Source: CAD feature listing. Evaluate the final solid. Frame: model axes, mm. A direction names the side the tool comes from. Coordinates: 2 decimals unless noted, no trailing zeros. Write each loop counter-clockwise with the first axis right and the second up, starting at its lowest first coordinate (ties: lowest second). Pieces come first, ordered by that corner, then holes. Notation, with made-up numbers: M 31.5,52.5 L 74.5,52.5 A18 ccw 74.5,81.5 Z; hole C 89,67 d2. An arc over 180 degrees is marked long. One line per item, written item: value. Start each with the question number.
Item 1: Cut plane C-C, the plane z = -15. Output: boundary loops of the cut face in (x, y), then the cut area to 3 significant figures.
Item 2: Mould query, pull axis X, two halves, no side actions, for faces 4 (the flat face through (-1, -1.524, -7)), 5 (the cylindrical face through (-41.86, 0.02, -7.84)), 6 (the cylindrical face through (-22.2, 0.02, -10.71)). Classes: released by +X, released by -X, zero draft, split by the parting line, or undercut.
Item 3: Pin query (flat end, axial travel): P1, Ø0.9, axis at x = 3, y = 1, coming from the -Z side; P2, Ø1, axis at x = -22, y = 1, coming from the -Z side. Return the tip coordinate at first contact, or that it passes through.
Item 4: Cut plane B-B, the plane x = 38. Output: boundary loops of the cut face in (y, z).
Item 5: Set-up query: faces 1 (the flat face through (17, 0, -9.901)), 2 (the cylindrical face through (51.045, -0.021, -4.914)), 3 (the flat face through (-48.217, 0.021, -4.079)). Return all of +Z, -Z, +X, -X, +Y, -Y with unobstructed straight access to the full face (end or side cutting, diameter ignored); none if empty.
Item 6: Cut plane D-D, the plane x = -33. Output: boundary loops of the cut face in (y, z).
Item 7: Cut plane A-A, the plane y = 0.1. Output: boundary loops of the cut face in (x, z).
Item 8: Ray query, L1, parallel to Z at x = 1.5, y = 0; L2, parallel to X at y = 0.9, z = -11.25; L3, parallel to X at y = 0.65, z = -16.5. Return the intervals inside material, ascending. Write a range as from..to.
```python
from build123d import *

# Parameters (mm, degrees)
F1_OUTLINE_DEPTH            = 1.524
F2_SLOT_DEPTH               = 58.881120617
F2_SLOT_DEPTH_BACK          = 58.881120617
F3A_HANDLEROUNDS_DEPTH      = 50.053367
F3A_HANDLEROUNDS_DEPTH_BACK = 11.2136936
F3B_ENDROUND_ANGLE          = 180
F4_RUNOUT_TOP_POS_ANGLE     = 90
F4_RUNOUT_BOT_POS_ANGLE     = 90
F4_RUNOUT_TOP_NEG_ANGLE     = 90
F4_RUNOUT_BOT_NEG_ANGLE     = 90


with BuildPart() as part:
    # SK_F1_Outline → F1_Outline (new, symmetric)
    with BuildSketch(Plane(origin=(0, 0, 0), x_dir=(1, 0, 0), z_dir=(0, 1, 0))):
        with BuildLine():
            Line((-34.3917778, 0), (50.053367, 0))
            ThreePointArc((50.053367, 0), (55.0037, 4.950333), (50.053367, 9.900666))
            Line((50.053367, 9.900666), (-17.8811936, 9.900666))
            ThreePointArc((-17.8811936, 9.900666), (-22.254213469, 10.732825234), (-26.01595, 13.1129786))
            ThreePointArc((-26.01595, 13.1129786), (-42.046618803, 17.559873613), (-54.849649, 6.9372734))
            ThreePointArc((-54.849649, 6.9372734), (-54.781279257, 5.257869905), (-53.4488136, 4.2333672))
            Line((-53.4488136, 4.2333672), (-49.0586522, 3.26009))
            Line((-49.0586522, 3.26009), (-47.3517722, 4.920488))
            Line((-47.3517722, 4.920488), (-48.8359196, 5.483987))
            ThreePointArc((-48.8359196, 5.483987), (-41.756588445, 7.823426138), (-35.8603296, 3.26009))
            Line((-35.8603296, 3.26009), (-34.3917778, 0))
        make_face()
    extrude(amount=F1_OUTLINE_DEPTH, both=True)

    # SK_F2_Slot → F2_Slot (cut, two sides: drawn at the far end of the back side and taken through both)
    with BuildSketch(Plane(origin=(0, 0, 0), x_dir=(1, 0, 0), z_dir=(0, 1, 0)).offset(-F2_SLOT_DEPTH_BACK)):
        with BuildLine():
            Line((48.7354118, 3.300222), (49.3954308, 3.300222))
            ThreePointArc((49.3954308, 3.300222), (51.0455418, 4.950333), (49.3954308, 6.600444))
            Line((49.3954308, 6.600444), (48.7354118, 6.600444))
            ThreePointArc((48.7354118, 6.600444), (47.0853008, 4.950333), (48.7354118, 3.300222))
        make_face()
    extrude(amount=F2_SLOT_DEPTH + F2_SLOT_DEPTH_BACK, mode=Mode.SUBTRACT)

    # SK_F3_StraightRounds → F3a_HandleRounds (cut, two sides: drawn at the far end of the back side and taken through both)
    with BuildSketch(Plane(origin=(0, 0, 0), x_dir=(0, 0, -1), z_dir=(1, 0, 0)).offset(-F3A_HANDLEROUNDS_DEPTH_BACK)):
        with BuildLine():
            Line((0, 1.127125), (-0.254, 1.127125))
            Line((-0.254, 1.127125), (-0.254, 1.778))
            Line((-0.254, 1.778), (0.396875, 1.778))
            Line((0.396875, 1.778), (0.396875, 1.524))
            ThreePointArc((0.396875, 1.524), (0.116241996, 1.407758004), (0, 1.127125))
        make_face()
        with BuildLine():
            Line((9.900666, 1.127125), (10.154666, 1.127125))
            Line((10.154666, 1.127125), (10.154666, 1.778))
            Line((10.154666, 1.778), (9.503791, 1.778))
            Line((9.503791, 1.778), (9.503791, 1.524))
            ThreePointArc((9.503791, 1.524), (9.784424004, 1.407758004), (9.900666, 1.127125))
        make_face()
        with BuildLine():
            Line((0, -1.127125), (-0.254, -1.127125))
            Line((-0.254, -1.127125), (-0.254, -1.778))
            Line((-0.254, -1.778), (0.396875, -1.778))
            Line((0.396875, -1.778), (0.396875, -1.524))
            ThreePointArc((0.396875, -1.524), (0.116241996, -1.407758004), (0, -1.127125))
        make_face()
        with BuildLine():
            Line((9.900666, -1.127125), (10.154666, -1.127125))
            Line((10.154666, -1.127125), (10.154666, -1.778))
            Line((10.154666, -1.778), (9.503791, -1.778))
            Line((9.503791, -1.778), (9.503791, -1.524))
            ThreePointArc((9.503791, -1.524), (9.784424004, -1.407758004), (9.900666, -1.127125))
        make_face()
    extrude(amount=F3A_HANDLEROUNDS_DEPTH + F3A_HANDLEROUNDS_DEPTH_BACK, mode=Mode.SUBTRACT)

    # SK_F3_EndRound → F3b_EndRound (revolve, symmetric, cut)
    with BuildSketch(Plane.XY.offset(-4.950333)) as f3b_endround_sk:
        with BuildLine():
            Line((55.0037, 1.127125), (55.2577, 1.127125))
            Line((55.2577, 1.127125), (55.2577, 1.778))
            Line((55.2577, 1.778), (54.606825, 1.778))
            Line((54.606825, 1.778), (54.606825, 1.524))
            ThreePointArc((54.606825, 1.524), (54.887458004, 1.407758004), (55.0037, 1.127125))
        make_face()
        with BuildLine():
            Line((55.0037, -1.127125), (55.2577, -1.127125))
            Line((55.2577, -1.127125), (55.2577, -1.778))
            Line((55.2577, -1.778), (54.606825, -1.778))
            Line((54.606825, -1.778), (54.606825, -1.524))
            ThreePointArc((54.606825, -1.524), (54.887458004, -1.407758004), (55.0037, -1.127125))
        make_face()
    revolve(axis=Axis((50.053367, -2.54, -4.950333), (0, 1, 0)), revolution_arc=F3B_ENDROUND_ANGLE / 2, mode=Mode.SUBTRACT)
    revolve(f3b_endround_sk.sketch, axis=Axis((50.053367, -2.54, -4.950333), (0, -1, 0)), revolution_arc=F3B_ENDROUND_ANGLE / 2, mode=Mode.SUBTRACT)

    # SK_F4_Runout1 → F4_Runout_Top_Pos (revolve, cut)
    with BuildSketch(Plane(origin=(0, 1.127125, 0), x_dir=(1, 0, 0), z_dir=(0, 1, 0))):
        Polygon((-11.2136936, 0), (-12.1460006, -0.164390878), (-12.1460006, -0.365125), (-11.2136936, -0.365125), align=None)
    revolve(axis=Axis((-9.9436936, 1.127125, -0.396875), (-1, 0, 0)), revolution_arc=F4_RUNOUT_TOP_POS_ANGLE, mode=Mode.SUBTRACT)

    # SK_F4_Runout2 → F4_Runout_Bot_Pos (revolve, cut)
    with BuildSketch(Plane(origin=(0, 1.127125, 0), x_dir=(1, 0, 0), z_dir=(0, 1, 0))):
        Polygon((-11.2136936, 9.900666), (-12.1460006, 10.065056878), (-12.1460006, 10.265791), (-11.2136936, 10.265791), align=None)
    revolve(axis=Axis((-9.9436936, 1.127125, -9.503791), (1, 0, 0)), revolution_arc=F4_RUNOUT_BOT_POS_ANGLE, mode=Mode.SUBTRACT)

    # SK_F4_Runout3 → F4_Runout_Top_Neg (revolve, cut)
    with BuildSketch(Plane(origin=(0, -1.127125, 0), x_dir=(1, 0, 0), z_dir=(0, 1, 0))):
        Polygon((-11.2136936, 0), (-12.1460006, -0.164390878), (-12.1460006, -0.365125), (-11.2136936, -0.365125), align=None)
    revolve(axis=Axis((-9.9436936, -1.127125, -0.396875), (1, 0, 0)), revolution_arc=F4_RUNOUT_TOP_NEG_ANGLE, mode=Mode.SUBTRACT)

    # SK_F4_Runout4 → F4_Runout_Bot_Neg (revolve, cut)
    with BuildSketch(Plane(origin=(0, -1.127125, 0), x_dir=(1, 0, 0), z_dir=(0, 1, 0))):
        Polygon((-11.2136936, 9.900666), (-12.1460006, 10.065056878), (-12.1460006, 10.265791), (-11.2136936, 10.265791), align=None)
    revolve(axis=Axis((-9.9436936, -1.127125, -9.503791), (-1, 0, 0)), revolution_arc=F4_RUNOUT_BOT_NEG_ANGLE, mode=Mode.SUBTRACT)


solid = part.part
```
From the geometry:
1. outline: M -48.16,-1.52 L -28.41,-1.52 L -28.41,1.52 L -48.16,1.52 Z
1. area: 60.2 mm²
2. face 4: zero draft
2. face 5: undercut
2. face 6: released by +X
3. P1: stops at z = -9.9
3. P2: stops at z = -10.83
4. outline: M -1.52,-9.5 A0.4 ccw -1.13,-9.9 L 1.13,-9.9 A0.4 ccw 1.52,-9.5 L 1.52,-0.4 A0.4 ccw 1.13,0 L -1.13,0 A0.4 ccw -1.52,-0.4 Z
5. face 1: -Z, +X, +Y, -Y
5. face 2: +Y, -Y
5. face 3: +Z, +Y, -Y
6. outline: M -1.52,-17.16 L 1.52,-17.16 L 1.52,0 L -1.52,0 Z
7. outline: M -54.85,-6.94 A17.96 ccw -26.02,-13.11 A11.91 cw -17.88,-9.9 L 50.05,-9.9 A4.95 ccw 50.05,0 L -34.39,0 L -35.86,-3.26 A7.94 cw -48.84,-5.48 L -47.35,-4.92 L -49.06,-3.26 L -53.45,-4.23 A1.98 ccw Z; hole M 48.74,-6.6 L 49.4,-6.6 A1.65 ccw 49.4,-3.3 L 48.74,-3.3 A1.65 ccw Z
8. L1: z = -9.9..0
8. L2: x = -52.28..-23.39
8. L3: x = -45.37..-31.2
